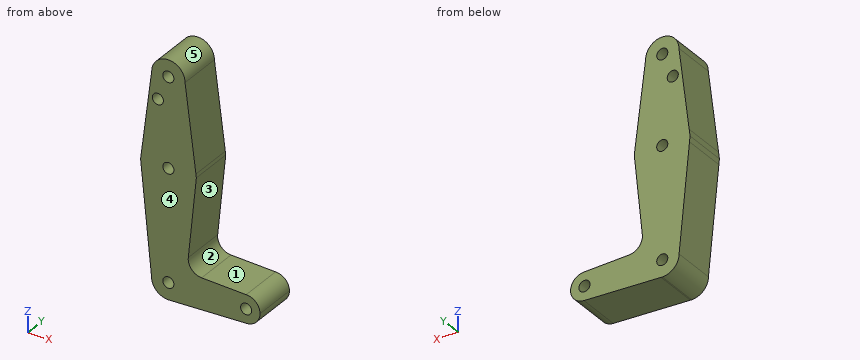
```python
from build123d import *

# Parameters (mm, degrees)
F0_R     = 3.175
F1_DEPTH = 25.4


with BuildPart() as f1:
    # F0 (on Front) → F1 (new body)
    with BuildSketch(Plane.XZ):
        with BuildLine():
            ThreePointArc((-9.602438, 0), (0, 9.602438), (9.602438, 0))
            ThreePointArc((9.602438, 0), (7.038529, -6.531916), (0.715959, -9.57571))
            Line((0.715959, -9.57571), (44.746117, -7.931975))
            ThreePointArc((44.746117, -7.931975), (36.513881, -0.148084), (44.45, 7.9375))
            Line((44.45, 7.9375), (18.991657, 8.894967))
            ThreePointArc((18.991657, 8.894967), (13.294448, 11.619044), (11.380335, 17.636931))
            Line((11.380335, 17.636931), (16.003576, 63.5))
            Line((16.003576, 63.5), (15.747457, 65.508289))
            ThreePointArc((15.747457, 65.508289), (15.843082, 64.506168), (15.875, 63.5))
            ThreePointArc((15.875, 63.5), (1.560545, 47.701889), (-15.56819, 60.394026))
            Line((-15.56819, 60.394026), (-9.602438, 0))
        make_face()
        with BuildLine():
            Line((-9.525, 114.3), (-15.386538, 67.407692))
            ThreePointArc((-15.386538, 67.407692), (0.966695, 79.34554), (15.747457, 65.508289))
            Line((15.747457, 65.508289), (9.525, 114.3))
            ThreePointArc((9.525, 114.3), (0, 104.775), (-9.525, 114.3))
        make_face()
        with Locations((-6.005472, 100.0252)):
            Circle(F0_R, mode=Mode.SUBTRACT)
        with BuildLine():
            Line((-15.875, 63.5), (-15.56819, 60.394026))
            ThreePointArc((-15.56819, 60.394026), (1.560545, 47.701889), (15.875, 63.5))
            ThreePointArc((15.875, 63.5), (15.843082, 64.506168), (15.747457, 65.508289))
            ThreePointArc((15.747457, 65.508289), (0.966695, 79.34554), (-15.386538, 67.407692))
            Line((-15.386538, 67.407692), (-15.875, 63.5))
        make_face()
        with Locations((0, 63.5)):
            Circle(F0_R, mode=Mode.SUBTRACT)
        with BuildLine():
            ThreePointArc((0.715959, -9.57571), (7.038529, -6.531916), (9.602438, 0))
            ThreePointArc((9.602438, 0), (0, 9.602438), (-9.602438, 0))
            ThreePointArc((-9.602438, 0), (-6.789949, -6.789949), (0, -9.602438))
            Line((0, -9.602438), (0.715959, -9.57571))
        make_face()
        Circle(F0_R, mode=Mode.SUBTRACT)
        with BuildLine():
            ThreePointArc((44.45, 7.9375), (36.513881, -0.148084), (44.746117, -7.931975))
            ThreePointArc((44.746117, -7.931975), (50.166395, -5.506972), (52.3875, 0))
            ThreePointArc((52.3875, 0), (50.06266, 5.61266), (44.45, 7.9375))
        make_face()
        with Locations((44.45, 0)):
            Circle(F0_R, mode=Mode.SUBTRACT)
        with BuildLine():
            ThreePointArc((9.525, 114.3), (0, 123.825), (-9.525, 114.3))
            ThreePointArc((-9.525, 114.3), (0, 104.775), (9.525, 114.3))
        make_face()
        with Locations((0, 114.3)):
            Circle(F0_R, mode=Mode.SUBTRACT)
    extrude(amount=F1_DEPTH)


solid = f1.part
```
Work out the finished part from the listing and answer in its coordinate system (mm). Face numbers are marked on the shaded views. A direction names the side the tool comes from. Coordinates: 2 decimals unless noted, no trailing zeros. Loops run counter-clockwise (first coordinate to the right, second up) from the corner with the lowest first, then second, coordinate; pieces in that order, holes last.
1) For the marked faces 1 and 2, determine the directions among +Z, -Z, +X, -X, +Y, -Y from which every point of the face is accessible in a straight line to the end or side of a thin tool.
Results:
face 1: +Z, +X, +Y, -Y
face 2: +X, +Y, -Y
2) Flat-ended cylindrical pins translate along their axes: pin 1 (6 mm diameter, centred on x = 38.5, y = -10.5, fed in from +Z); pin 2 (6 mm diameter, centred on x = 5, y = -23, fed in from -Z); pin 3 (6 mm diameter, centred on y = -14.5, z = 95.5, fed in from +X). Find the tip coordinate at first contact, or state that the pin passes through.
Results:
pin 1: stops at z = 8.27
pin 2: stops at z = -9.53
pin 3: stops at x = 12.31
3) Consider probe 1 along Z at (x, y) = (0, -14.25) (3 decimals); probe 2 along Z at (x, y) = (0.5, -8.75); probe 3 along Z at (x, y) = (45, -16.5). Determine where each line is inside the solid, lowest interval first.
Results:
probe 1: z = -9.602 to -3.175, 3.175 to 60.325, 66.675 to 111.125, 117.475 to 123.825
probe 2: z = -9.58 to -3.14, 3.14 to 60.36, 66.64 to 111.16, 117.44 to 123.81
probe 3: z = -7.92 to -3.13, 3.13 to 7.92
4) Section C-C (x = -5) is taken. Give the vertices of the cut face in (y, z), plus the area to 3 significant figures.
Results:
outline: (-25.4, -8.2) - (0, -8.2) - (0, 97.01) - (-25.4, 97.01) - close; (-25.4, 103.04) - (0, 103.04) - (0, 122.41) - (-25.4, 122.41) - close
area: 3,160 mm2
5) Section A-A (x = 46) is taken. Give the vertices of the cut face in (y, z).
Results:
outline: (-25.4, -7.78) - (0, -7.78) - (0, -2.77) - (-25.4, -2.77) - close; (-25.4, 2.77) - (0, 2.77) - (0, 7.78) - (-25.4, 7.78) - close
6) For a pull along Z with two mould halves and no side action, classify the marked faces 3, 4 and 5 as +Z half, -Z half, draft (parallel to the pull), parting line (faces both ways), or undercut.
Results:
face 3: undercut
face 4: draft
face 5: +Z half
7) Section B-B (y = -4.75) is taken. Give the number of separate pieces and of enclosed holes in the cut face, plus the area to 3 significant figures.
Results:
separate pieces: 1
enclosed holes: 5
area: 3,770 mm2
8) Section D-D (z = 53) is taken. Give the vertices of the cut face in (x, y).
Results:
outline: (-14.84, -25.4) - (14.95, -25.4) - (14.95, 0) - (-14.84, 0) - close
